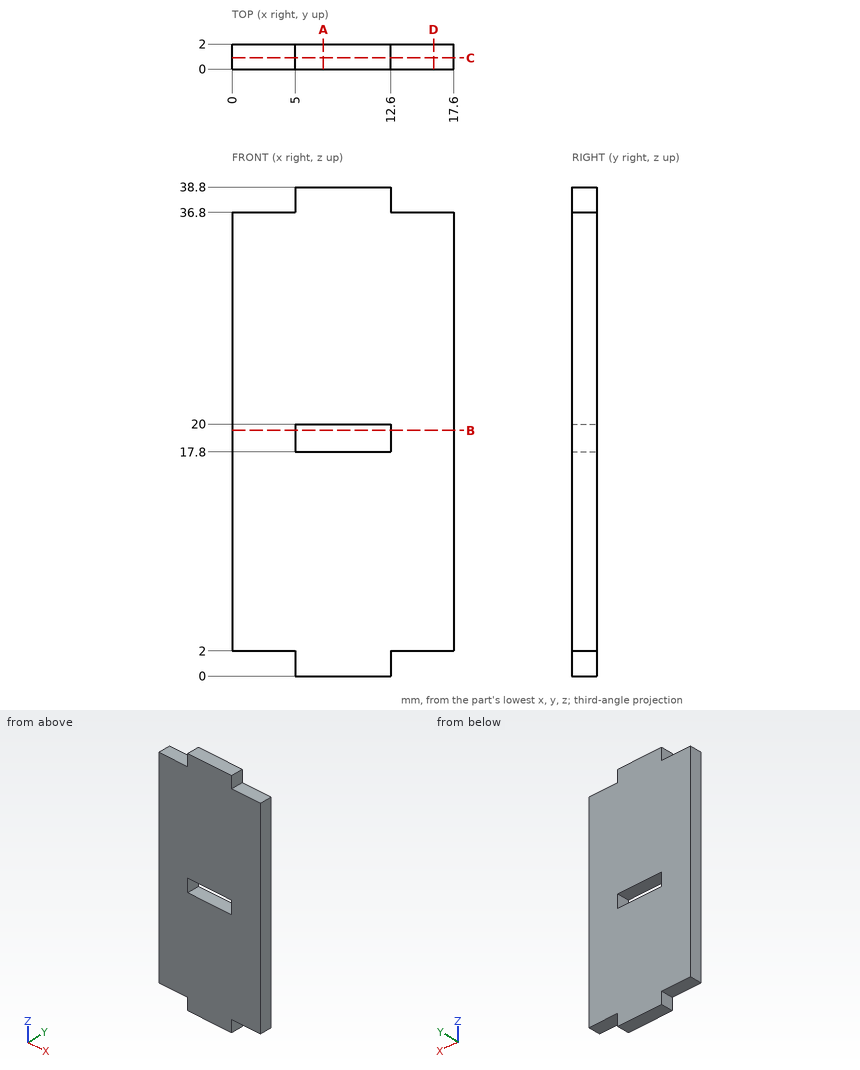
Could you check a few things on this drawing? It's one solid part, dimensions in mm from its lowest x, y, z. Round coordinates to 2 decimals unless told otherwise and drop trailing zeros. Order: outer loops, then holes, each group sorted by start corner. A loop starts at its lowest first (then second) coordinate and runs counter-clockwise, first axis right, second up. Notation, with made-up numbers: M -29,11 L -21,11 A17 ccw -21,26 Z; hole C 31,-4 d9. An arc over 180 degrees is marked long. Use a Markdown table: item, result.
1) Imagine slicing it at C-C (y = 0.9). List the corners of the cut face in (x, z) for me, then the cut area to 3 significant figures.
Geometry says:
| item | result |
|---|---|
| outline | M 0,2 L 5,2 L 5,0 L 12.6,0 L 12.6,2 L 17.6,2 L 17.6,36.8 L 12.6,36.8 L 12.6,38.8 L 5,38.8 L 5,36.8 L 0,36.8 Z; hole M 5,17.8 L 12.6,17.8 L 12.6,20 L 5,20 Z |
| area | 626 mm² |
2) Imagine slicing it at D-D (x = 16). List the corners of the cut face in (y, z) for me, then the cut area to 3 significant figures.
Geometry says:
| item | result |
|---|---|
| outline | M 0,2 L 2,2 L 2,36.8 L 0,36.8 Z |
| area | 69.6 mm² |
3) Imagine slicing it at B-B (z = 19.5). List the corners of the cut face in (x, y) for me.
Geometry says:
| item | result |
|---|---|
| outline | M 0,0 L 5,0 L 5,2 L 0,2 Z; M 12.6,0 L 17.6,0 L 17.6,2 L 12.6,2 Z |
4) Imagine slicing it at A-A (x = 7.25). List the corners of the cut face in (y, z) for me.
Geometry says:
| item | result |
|---|---|
| outline | M 0,0 L 2,0 L 2,17.8 L 0,17.8 Z; M 0,20 L 2,20 L 2,38.8 L 0,38.8 Z |
5) I'm going to push flat-ended pins straight in: P1, Ø0.6, axis at y = 1.5, z = 37.5, coming from the -X side; P2, Ø1, axis at x = 14, y = 1.5, coming from the +Z side; P3, Ø3, axis at x = 12.5, z = 19, coming from the -Y side; P4, Ø1, axis at x = 3, y = 0.5, coming from the -Z side. Where does each tip first touch, or does it pass through?
Geometry says:
| item | result |
|---|---|
| P1 | stops at x = 5 |
| P2 | stops at z = 36.8 |
| P3 | stops at y = 0 |
| P4 | stops at z = 2 |
6) If I drill on line 1 along Z through (x, y) = (11, 1.3); line 2 along X through (y, z) = (1.4, 19); line 3 along Z through (x, y) = (4.5, 1.25), over which ranges is the centre line in solid material (lowest first)?
Geometry says:
| item | result |
|---|---|
| line 1 | z = 0 to 17.8, 20 to 38.8 |
| line 2 | x = 0 to 5, 12.6 to 17.6 |
| line 3 | z = 2 to 36.8 |
